The model under review builds one solid part; all positions refer to its coordinate system, in mm. A direction names the side the tool comes from. Round coordinates to 2 decimals unless told otherwise and drop trailing zeros. Order: outer loops, then holes, each group sorted by start corner. A loop starts at its lowest first (then second) coordinate and runs counter-clockwise, first axis right, second up. Notation, with made-up numbers: (24.5, 19.25) - (39.5, 19.25) arc R35 ccw to (39.5, 58.25) - close; hole circle Ø11 at (87, -29.5). An arc over 180 degrees is marked (long way). One line per question, with ' | ' between items. Start each with the question number.
Item 1: Add section B-B on z = 6. State the section outline as (x, y) points, and give its area (3 significant figures).
Item 2: Insertion check: pin 1 Ø6 at (x, y) = (-21, -13.5) entering from +Z; pin 2 Ø2.5 at (x, y) = (-14.5, -16) entering from +Z; pin 3 Ø1.5 at (x, y) = (13, -9) entering from +Z. Each pin has a flat end and moves straight along its axis. Give the tip position at first contact, or say it passes through.
Item 3: Tool access review of faces 1 (the face through (0, 1, -8.468)), 2 (the face through (23, -14, 5)), 3 (the face through (20.49, -12.74, 8.7)): name each direction out of +Z, -Z, +X, -X, +Y, -Y from which nothing blocks a thin tool from reaching the whole face with its end or side.
Item 4: Add section C-C on y = -17. State the section outline as (x, z) points, and give its area (3 significant figures).
Item 5: Draft analysis for pull direction Y (two halves, no side actions). For faces 4 (the face through (-16.94, 0.76, -22.71)), 5 (the face through (19.75, -6, 9)), 6 (the face through (21.21, -25.46, 8.7)), state which applies: +Y half, -Y half, draft (parallel to the pull), parting line (faces both ways), or undercut.
Item 6: Add section A-A on y = -25. State the section outline as (x, z) points.
Item 7: For L1, parallel to X at y = -7, z = 7.5; L2, parallel to Z at x = 21, y = -4.5; L3, parallel to Y at x = -19, z = 12, list the stretches that pass through material, from the lowest coordinate up. Write a range as [from, to].
Item 8: Add section D-D on x = -1.5. State the section outline as (y, z) points, and give its area (3 significant figures).
from build123d import *

# Parameters (mm, degrees)
SKETCH1_W           = 42.5
SKETCH1_H           = 44.5
BOSS_EXTRUDE1_DEPTH = 2
BOSS_EXTRUDE2_START = -27.25
BOSS_EXTRUDE2_DEPTH = 7.5
BOSS_EXTRUDE3_START = -5
BOSS_EXTRUDE3_DEPTH = 5
CUT_EXTRUDE3_DEPTH  = 5
CHAMFER1_SIZE       = 1.15
FILLET1_R           = 1


with BuildPart() as part:
    # Sketch1 → Boss-Extrude1 (new body)
    with BuildSketch(Plane(origin=(0, 0, 0), x_dir=(1, 0, 0), z_dir=(0, 1, 0))):
        Rectangle(SKETCH1_W, SKETCH1_H)
    extrude(amount=BOSS_EXTRUDE1_DEPTH)

    # Sketch2 → Boss-Extrude2 (add)
    with BuildSketch(Plane(origin=(0, 0, -22.25), x_dir=(-1, 0, 0), z_dir=(0, 0, -1)).offset(BOSS_EXTRUDE2_START)):
        Polygon((21.25, -22.5), (18.25, -22.5), (24.25, -28.5), (26.25, -28.5), (26.25, -18), (26.25, -6.660254038), (21.25, 2), (21.25, 0), (19.75, 0), (19.75, -12), (21.25, -13.5), align=None)
    boss_extrude2 = extrude(amount=-BOSS_EXTRUDE2_DEPTH)

    # Mirror1: Boss-Extrude2 across plane
    add(boss_extrude2.mirror(Plane(origin=(0, 0, 0), x_dir=(0, 0, 1), z_dir=(1, 0, 0))))

    # Sketch4 → Boss-Extrude3 (add)
    with BuildSketch(Plane(origin=(21.25, 0, 0), x_dir=(0, 0, -1), z_dir=(1, 0, 0)).offset(BOSS_EXTRUDE3_START)):
        Polygon((27.25, -6.660254038), (27.25, -28.5), (25.25, -28.5), (19.25, -22.5), (22.25, -22.5), (22.25, -13.5), (20.75, -12), (20.75, 0), (22.25, 0), (22.25, 2), align=None)
    boss_extrude3 = extrude(amount=-BOSS_EXTRUDE3_DEPTH)

    # Mirror2: Boss-Extrude3 across plane
    add(boss_extrude3.mirror(Plane(origin=(0, 0, 0), x_dir=(0, 0, 1), z_dir=(1, 0, 0))))

    # Sketch5 → Cut-Extrude3 (cut)
    with BuildSketch(Plane(origin=(0, 2, 0), x_dir=(1, 0, 0), z_dir=(0, 1, 0))):
        with BuildLine():
            ThreePointArc((0, -9.063025703), (-10.875563664, -10.802203854), (-21.25, -14.5))
            Line((-21.25, -14.5), (-21.25, -22.25))
            Line((-21.25, -22.25), (21.25, -22.25))
            Line((21.25, -22.25), (21.25, -14.5))
            ThreePointArc((21.25, -14.5), (10.875563664, -10.802203854), (0, -9.063025703))
        make_face()
        with BuildLine():
            Line((-21.25, 22.25), (-21.25, -3))
            add(Edge.make_bspline(
                [(-18.25, 22.25), (-16.81830639, 16.418600695), (-0.036255197, -2.877473786), (-21.25, -3)],
                knots=[0, 0, 0, 0, 1, 1, 1, 1], degree=3))
            Line((-18.25, 22.25), (-21.25, 22.25))
        make_face()
        with BuildLine():
            Line((-2.5, 8.468152214), (2.5, 8.468152214))
            ThreePointArc((2.5, 8.468152214), (7.249445146, 14.685907684), (9.25, 22.25))
            Line((9.25, 22.25), (-9.25, 22.25))
            ThreePointArc((-9.25, 22.25), (-7.249445146, 14.685907684), (-2.5, 8.468152214))
        make_face()
        with BuildLine():
            add(Edge.make_bspline(
                [(18.25, 22.25), (16.81830639, 16.418600695), (0.036255197, -2.877473786), (21.25, -3)],
                knots=[0, 0, 0, 0, 1, 1, 1, 1], degree=3))
            Line((21.25, -3), (21.25, 22.25))
            Line((21.25, 22.25), (18.25, 22.25))
        make_face()
    extrude(amount=-CUT_EXTRUDE3_DEPTH, mode=Mode.SUBTRACT)

    # Chamfer1
    chamfer1_edges = [part.edges().sort_by_distance(p)[0] for p in [
        (-11.25, 1, -22.25),
        (-21.25, 1, 12.5),
        (-21.25, 1, 5),
        (21.25, 1, 5),
        (21.25, 1, 12.5),
        (11.25, 1, -22.25),
        (16.25, 1, -22.25),
        (-16.25, 1, -22.25),
    ]]
    chamfer(chamfer1_edges, length=CHAMFER1_SIZE)

    # Fillet1
    # the kernel refuses this fillet: 1 mm, written as the material it takes off along each edge
    with BuildSketch(Plane(origin=(-21.25, 4.391127169, 3), x_dir=(0, 0, 1), z_dir=(0, -1, 0))) as fillet1_piece_1:
        with BuildLine():
            CenterArc((0.980089216, -0.991502292), FILLET1_R, 97.474747775, 80.505389302)
            Line((-0.019289453, -0.956256336), (-0.039277026, -0.955551417))
            ThreePointArc((-0.039277026, -0.955551417), (-0.026119359, -0.477798689), (-0.019999666, 0.000115514))
            Line((-0.019999666, 0.000115514), (0, 0.02))
            ThreePointArc((0, 0.02), (0.425, 0.02), (0.847398216, 0.019830046))
            Line((0.847398216, 0.019830046), (0.85, 0))
        make_face()
    extrude(amount=6.782254339, mode=Mode.SUBTRACT)
    with BuildSketch(Plane(origin=(-18.25, 5.318683713, -22.25), x_dir=(0.3309539081211192, 0, 0.9436469205690006), z_dir=(0, -1, 0))) as fillet1_piece_2:
        with BuildLine():
            CenterArc((1.261964238, -0.997851962), FILLET1_R, 86.243906852, 82.467431806)
            Line((0.281310822, -0.802099882), (0.261697754, -0.798184841))
            ThreePointArc((0.261697754, -0.798184841), (0.121782473, -0.407669019), (-0.018872938, -0.006619078))
            Line((-0.018872938, -0.006619078), (-0.001928232, 0.019906831))
            ThreePointArc((-0.001928232, 0.019906831), (0.664077557, 0.04586364), (1.32878367, 0.019957039))
            Line((1.32878367, 0.019957039), (1.327473485, 0))
        make_face()
    extrude(amount=8.637367425, mode=Mode.SUBTRACT)
    with BuildSketch(Plane(origin=(-9.25, 4.236352912, -22.25), x_dir=(-1, 0, 0), z_dir=(0, -1, 0))) as fillet1_piece_3:
        with BuildLine():
            CenterArc((0.919243583, -0.997599783), FILLET1_R, 93.970542278, 79.932192876)
            Line((-0.075099433, -0.891383179), (-0.094986293, -0.889258846))
            ThreePointArc((-0.094986293, -0.889258846), (-0.052494869, -0.444432453), (-0.01996196, 0.001232949))
            Line((-0.01996196, 0.001232949), (0, 0.02))
            ThreePointArc((0, 0.02), (0.425, 0.02), (0.848615128, 0.019951996))
            Line((0.848615128, 0.019951996), (0.85, 0))
        make_face()
    extrude(amount=6.472705825, mode=Mode.SUBTRACT)
    with BuildSketch(Plane(origin=(9.25, 4.236352912, -22.25), x_dir=(-0.08395302082723771, 0, 0.9964697136862621), z_dir=(0, -1, 0))) as fillet1_piece_4:
        with BuildLine():
            CenterArc((0.916904694, -0.999749905), FILLET1_R, 91.281442663, 79.932192876)
            Line((-0.071360068, -0.846999257), (-0.091125363, -0.843944244))
            ThreePointArc((-0.091125363, -0.843944244), (-0.055609428, -0.421820568), (-0.019929394, 0.00167906))
            Line((-0.019929394, 0.00167906), (0.000447271, 0.019994998))
            ThreePointArc((0.000447271, 0.019994998), (0.447270582, 0.0149981), (0.894093894, 0.019994998))
            Line((0.894093894, 0.019994998), (0.894541165, 0))
        make_face()
    extrude(amount=6.472705825, mode=Mode.SUBTRACT)
    with BuildSketch(Plane(origin=(18.25, 5.318683713, -22.25), x_dir=(-1, 0, 0), z_dir=(0, -1, 0))) as fillet1_piece_5:
        with BuildLine():
            CenterArc((1.359271928, -0.860605661), FILLET1_R, 120.615345392, 82.467431806)
            Line((0.439332538, -1.252666266), (0.42093375, -1.260507478))
            ThreePointArc((0.42093375, -1.260507478), (0.17649998, -0.641833493), (-0.019423176, -0.004768673))
            Line((-0.019423176, -0.004768673), (0, 0.02))
            ThreePointArc((0, 0.02), (0.425, 0.02), (0.839814561, 0.017212113))
            Line((0.839814561, 0.017212113), (0.85, 0))
        make_face()
    extrude(amount=8.637367425, mode=Mode.SUBTRACT)
    with BuildSketch(Plane(origin=(21.25, 4.391127169, 3), x_dir=(-0.9997966104440278, 0, -0.020167740196489006), z_dir=(0, -1, 0))) as fillet1_piece_6:
        with BuildLine():
            CenterArc((0.971534447, -0.999886236), FILLET1_R, 90.864258181, 80.505389302)
            Line((-0.017142579, -0.849827119), (-0.03691612, -0.846825937))
            ThreePointArc((-0.03691612, -0.846825937), (-0.028567222, -0.424510205), (-0.019995932, 0.000403355))
            Line((-0.019995932, 0.000403355), (0.000287858, 0.019997928))
            ThreePointArc((0.000287858, 0.019997928), (0.478228278, 0.016477927), (0.956149196, 0.019997725))
            Line((0.956149196, 0.019997725), (0.956450868, 0))
        make_face()
    extrude(amount=6.782254339, mode=Mode.SUBTRACT)
    with BuildSketch(Plane(origin=(21.25, 5.281576595, 14.5), x_dir=(0, 0, -1), z_dir=(0, -1, 0))) as fillet1_piece_7:
        with BuildLine():
            CenterArc((1.455421085, -0.79590534), FILLET1_R, 127.259148945, 76.371212097)
            Line((0.539270629, -1.196739897), (0.52094762, -1.204756588))
            ThreePointArc((0.52094762, -1.204756588), (0.254673852, -0.605111829), (-0.018143252, -0.008415604))
            Line((-0.018143252, -0.008415604), (0, 0.02))
            ThreePointArc((0, 0.02), (0.425, 0.02), (0.837891578, 0.015918107))
            Line((0.837891578, 0.015918107), (0.85, 0))
        make_face()
    extrude(amount=8.56315319, mode=Mode.SUBTRACT)
    with BuildSketch(Plane(origin=(-21.25, 5.281576595, 14.5), x_dir=(0, 0, -1), z_dir=(0, -1, 0))) as fillet1_piece_8:
        with BuildLine():
            CenterArc((1.455421085, 0.79590534), FILLET1_R, 156.369638958, 76.371212097)
            Line((0.539270629, 1.196739897), (0.52094762, 1.204756588))
            ThreePointArc((0.52094762, 1.204756588), (0.254673852, 0.605111829), (-0.018143252, 0.008415604))
            Line((-0.018143252, 0.008415604), (0, -0.02))
            ThreePointArc((0, -0.02), (0.425, -0.02), (0.837891578, -0.015918107))
            Line((0.837891578, -0.015918107), (0.85, 0))
        make_face()
    extrude(amount=8.56315319, mode=Mode.SUBTRACT)


solid = part.part
Determined:
1) outline: (-26.25, -28.5) - (-24.25, -28.5) - (-18.25, -22.5) - (-21.25, -22.5) - (-21.25, -13.5) - (-19.75, -12) - (-19.75, 0) - (19.75, 0) - (19.75, -12) - (21.25, -13.5) - (21.25, -22.5) - (18.25, -22.5) - (24.25, -28.5) - (26.25, -28.5) - (26.25, -6.66) - (21.25, 2) - (-21.25, 2) - (-26.25, -6.66) - close | area: 385 mm2
2) pin 1: z = 12.5 | pin 2: z = -22.25 | pin 3: z = -20.75
3) face 1: -Z, +Y, -Y | face 2: -Z, +X, -X, -Y | face 3: +Z, -Z
4) outline: (-26.25, 5) - (-21.25, 5) - (-21.25, 12.5) - (-26.25, 12.5) - close; (-16.25, -27.25) - (-11.25, -27.25) - (-11.25, -22.25) - (-16.25, -22.25) - close; (11.25, -27.25) - (16.25, -27.25) - (16.25, -22.25) - (11.25, -22.25) - close; (21.25, 5) - (26.25, 5) - (26.25, 12.5) - (21.25, 12.5) - close | area: 125 mm2
5) face 4: draft | face 5: undercut | face 6: -Y half
6) outline: (-26.25, 5) - (-20.75, 5) - (-20.75, 12.5) - (-26.25, 12.5) - close; (-16.25, -27.25) - (-11.25, -27.25) - (-11.25, -21.75) - (-16.25, -21.75) - close; (11.25, -27.25) - (16.25, -27.25) - (16.25, -21.75) - (11.25, -21.75) - close; (20.75, 5) - (26.25, 5) - (26.25, 12.5) - (20.75, 12.5) - close
7) L1: [-26.25, -19.75], [19.75, 26.25] | L2: [5, 12.5] | L3: [-23.25, -22.5], [0, 2]
8) outline: (0, -8.47) - (2, -8.47) - (2, 9.18) - (0, 9.18) - close | area: 35.3 mm2
